from build123d import *

# Parameters (mm, degrees)
SKETCH2_R            = 25.79
BOSS_EXTRUDE2_DEPTH  = 358
BOSS_EXTRUDE10_DEPTH = 358
SKETCH18_R           = 25.79
CUT_EXTRUDE5_DEPTH   = 358


with BuildPart() as part:
    # Sketch2 → Boss-Extrude2 (new body)
    with BuildSketch(Plane(origin=(0, 0, 0), x_dir=(0, 0, -1), z_dir=(1, 0, 0))):
        with Locations(Location((0, 0, 0), (0, 0, 180))):
            Circle(SKETCH2_R)
        with BuildLine():
            Line((9.521706212, 3.055668636), (16.449909442, 7.055668636))
            Line((16.449909442, 7.055668636), (14.335343, 10.718205149))
            Line((14.335343, 10.718205149), (7.40713977, 6.718205149))
            ThreePointArc((7.40713977, 6.718205149), (5, 8.660254038), (2.114566442, 9.773873785))
            Line((2.114566442, 9.773873785), (2.114566442, 17.773873785))
            Line((2.114566442, 17.773873785), (-2.114566442, 17.773873785))
            Line((-2.114566442, 17.773873785), (-2.114566442, 9.773873785))
            ThreePointArc((-2.114566442, 9.773873785), (-5, 8.660254038), (-7.40713977, 6.718205149))
            Line((-7.40713977, 6.718205149), (-14.335343, 10.718205149))
            Line((-14.335343, 10.718205149), (-16.449909442, 7.055668636))
            Line((-16.449909442, 7.055668636), (-9.521706212, 3.055668636))
            ThreePointArc((-9.521706212, 3.055668636), (-10, 0), (-9.521706212, -3.055668636))
            Line((-9.521706212, -3.055668636), (-16.449909442, -7.055668636))
            Line((-16.449909442, -7.055668636), (-14.335343, -10.718205149))
            Line((-14.335343, -10.718205149), (-7.40713977, -6.718205149))
            ThreePointArc((-7.40713977, -6.718205149), (-5, -8.660254038), (-2.114566442, -9.773873785))
            Line((-2.114566442, -9.773873785), (-2.114566442, -17.773873785))
            Line((-2.114566442, -17.773873785), (2.114566442, -17.773873785))
            Line((2.114566442, -17.773873785), (2.114566442, -9.773873785))
            ThreePointArc((2.114566442, -9.773873785), (5, -8.660254038), (7.40713977, -6.718205149))
            Line((7.40713977, -6.718205149), (14.335343, -10.718205149))
            Line((14.335343, -10.718205149), (16.449909442, -7.055668636))
            Line((16.449909442, -7.055668636), (9.521706212, -3.055668636))
            ThreePointArc((9.521706212, -3.055668636), (10, 0), (9.521706212, 3.055668636))
        make_face(mode=Mode.SUBTRACT)
    extrude(amount=BOSS_EXTRUDE2_DEPTH)

    # Sketch10 → Boss-Extrude10 (add)
    with BuildSketch(Plane.ZY):
        with BuildLine():
            Line((-7.114566442, -13.205413448), (-7.114566442, -17.773873785))
            ThreePointArc((-7.114566442, -17.773873785), (-5.650100348, -21.309407691), (-2.114566442, -22.773873785))
            Line((-2.114566442, -22.773873785), (2.114566442, -22.773873785))
            ThreePointArc((2.114566442, -22.773873785), (5.650100348, -21.309407691), (7.114566442, -17.773873785))
            Line((7.114566442, -17.773873785), (7.114566442, -13.205413448))
            ThreePointArc((7.114566442, -13.205413448), (7.5, -12.990381057), (7.878940293, -12.764102))
            Line((7.878940293, -12.764102), (11.835343, -15.048332168))
            ThreePointArc((11.835343, -15.048332168), (15.629438226, -15.547834281), (18.665470019, -13.218205149))
            Line((18.665470019, -13.218205149), (20.780036461, -9.555668636))
            ThreePointArc((20.780036461, -9.555668636), (21.279538574, -5.76157341), (18.949909442, -2.725541617))
            Line((18.949909442, -2.725541617), (14.993506735, -0.441311448))
            ThreePointArc((14.993506735, -0.441311448), (15, 0), (14.993506735, 0.441311448))
            Line((14.993506735, 0.441311448), (18.949909442, 2.725541617))
            ThreePointArc((18.949909442, 2.725541617), (21.279538574, 5.76157341), (20.780036461, 9.555668636))
            Line((20.780036461, 9.555668636), (18.665470019, 13.218205149))
            ThreePointArc((18.665470019, 13.218205149), (15.629438226, 15.547834281), (11.835343, 15.048332168))
            Line((11.835343, 15.048332168), (7.878940293, 12.764102))
            ThreePointArc((7.878940293, 12.764102), (7.5, 12.990381057), (7.114566442, 13.205413448))
            Line((7.114566442, 13.205413448), (7.114566442, 17.773873785))
            ThreePointArc((7.114566442, 17.773873785), (5.650100348, 21.309407691), (2.114566442, 22.773873785))
            Line((2.114566442, 22.773873785), (-2.114566442, 22.773873785))
            ThreePointArc((-2.114566442, 22.773873785), (-5.650100348, 21.309407691), (-7.114566442, 17.773873785))
            Line((-7.114566442, 17.773873785), (-7.114566442, 13.205413448))
            ThreePointArc((-7.114566442, 13.205413448), (-7.5, 12.990381057), (-7.878940293, 12.764102))
            Line((-7.878940293, 12.764102), (-11.835343, 15.048332168))
            ThreePointArc((-11.835343, 15.048332168), (-15.629438226, 15.547834281), (-18.665470019, 13.218205149))
            Line((-18.665470019, 13.218205149), (-20.780036461, 9.555668636))
            ThreePointArc((-20.780036461, 9.555668636), (-21.279538574, 5.76157341), (-18.949909442, 2.725541617))
            Line((-18.949909442, 2.725541617), (-14.993506735, 0.441311448))
            ThreePointArc((-14.993506735, 0.441311448), (-15, 0), (-14.993506735, -0.441311448))
            Line((-14.993506735, -0.441311448), (-18.949909442, -2.725541617))
            ThreePointArc((-18.949909442, -2.725541617), (-21.279538574, -5.76157341), (-20.780036461, -9.555668636))
            Line((-20.780036461, -9.555668636), (-18.665470019, -13.218205149))
            ThreePointArc((-18.665470019, -13.218205149), (-15.629438226, -15.547834281), (-11.835343, -15.048332168))
            Line((-11.835343, -15.048332168), (-7.878940293, -12.764102))
            ThreePointArc((-7.878940293, -12.764102), (-7.5, -12.990381057), (-7.114566442, -13.205413448))
        make_face()
    extrude(amount=BOSS_EXTRUDE10_DEPTH)

    # Sketch18 → Cut-Extrude5 (cut)
    with BuildSketch(Plane.ZY):
        Circle(SKETCH18_R)
    extrude(amount=-CUT_EXTRUDE5_DEPTH, mode=Mode.SUBTRACT)


solid = part.part
Check sheet for the modelled part. Datum: model origin and axes. Units: mm. Round coordinates to 2 decimals unless told otherwise and drop trailing zeros. Return JSON: item names as keys, results as strings.
Q1. Depth check by flat-ended pin: P1, Ø1, axis at x = -99.5, z = -13, coming from the -Y side; P2, Ø3, axis at x = -112, z = -9.5, coming from the -Y side; P3, Ø12, axis at x = -193, y = -18, coming from the +Z side; P4, Ø1, axis at y = 18, z = 14.5, coming from the -X side. Enter the tip coordinate at first touch or a pass-through.
Returned:
{"P1": "stops at y = -15.65", "P2": "stops at y = -14.57", "P3": "stops at z = 19.37", "P4": "passes through"}
Q2. Draft check along Z on faces 1 (the flat face through (-358, 0, 0)), 2 (the cylindrical face through (-176.494, -5.815, 21.293)), 3 (the cylindrical face through (-176.49, -15.56, 15.58)). Enter one of: released by +Z, released by -Z, zero draft, split by the parting line, or undercut.
Returned:
{"face 1": "zero draft", "face 2": "released by +Z", "face 3": "undercut"}
Q3. Scan lines: L1, parallel to Z at x = -318, y = 13.5; L2, parallel to Z at x = -108, y = 13; L3, parallel to Z at x = -177, y = -16. Record each from-to range of solid material in increasing order. Write a range as from..to.
Returned:
{"L1": "z = -18.49..-9.15, -7.11..7.11, 9.15..18.49", "L2": "z = -18.79..-8.29, -7.48..7.48, 8.29..18.79", "L3": "z = -7.11..7.11"}
